from build123d import *

# Parameters (mm, degrees)
SKETCH1_W                                           = 65
SKETCH1_H                                           = 75
BOSS_EXTRUDE1_DEPTH                                 = 10
SKETCH2_W                                           = 5
SKETCH2_H                                           = 75
BOSS_EXTRUDE2_DEPTH                                 = 15
CUT_EXTRUDE1_DEPTH                                  = 109
CUT_EXTRUDE3_DEPTH                                  = 6.2
CUT_EXTRUDE4_DEPTH                                  = 48.4
CBORE_FOR_M6_HEX_SOCKET_HEAD_CAP_SCREW1_D           = 6.6
CBORE_FOR_M6_HEX_SOCKET_HEAD_CAP_SCREW1_CBORE_D     = 11
CBORE_FOR_M6_HEX_SOCKET_HEAD_CAP_SCREW1_CBORE_DEPTH = 6.2
BOSS_EXTRUDE3_START                                 = 5
SKETCH9_W                                           = 25
SKETCH9_H                                           = 75
BOSS_EXTRUDE3_DEPTH                                 = 5
CHAMFER1_SIZE                                       = 1.5


with BuildPart() as part:
    # Sketch1 → Boss-Extrude1 (new body)
    with BuildSketch(Plane.XY):
        Rectangle(SKETCH1_W, SKETCH1_H)
    extrude(amount=BOSS_EXTRUDE1_DEPTH)

    # Sketch2 → Boss-Extrude2 (add)
    with BuildSketch(Plane(origin=(0, 0, 0), x_dir=(-1, 0, 0), z_dir=(0, 0, -1))):
        with Locations((-30, 0)):
            Rectangle(SKETCH2_W, SKETCH2_H)
        with Locations((30, 0)):
            Rectangle(SKETCH2_W, SKETCH2_H)
    extrude(amount=BOSS_EXTRUDE2_DEPTH)

    # Sketch3 → Cut-Extrude1 (cut)
    with BuildSketch(Plane.ZY.offset(32.5)):
        with BuildLine():
            Line((-4.75, 30), (-4.75, -30))
            ThreePointArc((-4.75, -30), (-7.5, -32.75), (-10.25, -30))
            Line((-10.25, -30), (-10.25, 30))
            ThreePointArc((-10.25, 30), (-7.5, 32.75), (-4.75, 30))
        make_face()
    extrude(amount=-CUT_EXTRUDE1_DEPTH, mode=Mode.SUBTRACT)

    # Sketch4 → Cut-Extrude3 (cut)
    with BuildSketch(Plane(origin=(0, 0, 0), x_dir=(-1, 0, 0), z_dir=(0, 0, -1))):
        with BuildLine():
            ThreePointArc((-23.364355515, 19.605022095), (-22.686442931, 11.856445805), (-14.937866641, 12.534358389))
            ThreePointArc((-14.937866641, 12.534358389), (0, 19.5), (14.937866641, 12.534358389))
            ThreePointArc((14.937866641, 12.534358389), (22.686442931, 11.856445805), (23.364355515, 19.605022095))
            ThreePointArc((23.364355515, 19.605022095), (0, 30.5), (-23.364355515, 19.605022095))
        make_face()
    extrude(amount=-CUT_EXTRUDE3_DEPTH, mode=Mode.SUBTRACT)

    # Sketch5 → Cut-Extrude4 (cut)
    with BuildSketch(Plane(origin=(0, 0, 0), x_dir=(-1, 0, 0), z_dir=(0, 0, -1))):
        with BuildLine():
            ThreePointArc((-21.67905774, 18.190889354), (-21.27231019, 13.54174358), (-16.623164416, 13.94849113))
            ThreePointArc((-16.623164416, 13.94849113), (0, 21.7), (16.623164416, 13.94849113))
            ThreePointArc((16.623164416, 13.94849113), (21.27231019, 13.54174358), (21.67905774, 18.190889354))
            ThreePointArc((21.67905774, 18.190889354), (0, 28.3), (-21.67905774, 18.190889354))
        make_face()
    extrude(amount=-CUT_EXTRUDE4_DEPTH, mode=Mode.SUBTRACT)

    # CBORE for M6 Hex Socket Head Cap Screw1 (through all)
    with Locations(Plane(origin=(0, 0, 0), x_dir=(-1, 0, 0), z_dir=(0, 0, -1))):
        with Locations((0, 0)):
            CounterBoreHole(CBORE_FOR_M6_HEX_SOCKET_HEAD_CAP_SCREW1_D / 2, CBORE_FOR_M6_HEX_SOCKET_HEAD_CAP_SCREW1_CBORE_D / 2, CBORE_FOR_M6_HEX_SOCKET_HEAD_CAP_SCREW1_CBORE_DEPTH)

    # Sketch9 → Boss-Extrude3 (add)
    with BuildSketch(Plane.ZY.offset(32.5).offset(BOSS_EXTRUDE3_START)):
        with Locations((-2.5, 0)):
            Rectangle(SKETCH9_W, SKETCH9_H)
        with BuildLine():
            Line((-4.75, 30), (-4.75, -30))
            ThreePointArc((-4.75, -30), (-7.5, -32.75), (-10.25, -30))
            Line((-10.25, -30), (-10.25, 30))
            ThreePointArc((-10.25, 30), (-7.5, 32.75), (-4.75, 30))
        make_face(mode=Mode.SUBTRACT)
    boss_extrude3 = extrude(amount=-BOSS_EXTRUDE3_DEPTH)

    # Mirror1: Boss-Extrude3 across plane
    add(boss_extrude3.mirror(Plane.ZY))

    # Chamfer1
    chamfer1_edges = [part.edges().sort_by_distance(p)[0] for p in [
        (-37.5, 0, -15),
        (-37.5, -37.5, -2.5),
        (-37.5, 0, 10),
        (-37.5, 37.5, -2.5),
        (37.5, 0, -15),
        (37.5, 37.5, -2.5),
        (37.5, 0, 10),
        (37.5, -37.5, -2.5),
        (0, -37.5, 10),
        (32.5, -37.5, -15),
        (32.5, 37.5, -15),
        (-32.5, 37.5, -15),
        (-32.5, -37.5, -15),
        (0, 37.5, 10),
    ]]
    chamfer(chamfer1_edges, length=CHAMFER1_SIZE)


solid = part.part
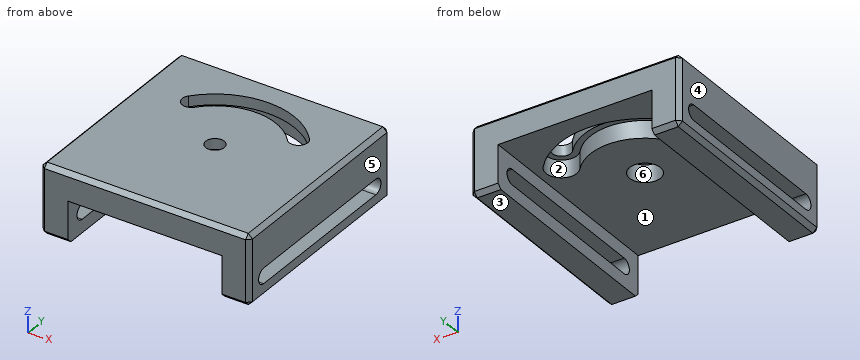
Check sheet for the modelled part. Datum: model origin and axes. Units: mm. Face numbers are marked on the shaded views. A direction names the side the tool comes from. Give positions to 0.01 mm unless a question says otherwise; leave off trailing zeros. Write each loop counter-clockwise with the first axis right and the second up, starting at its lowest first coordinate (ties: lowest second). Pieces come first, ordered by that corner, then holes. Notation, with made-up numbers: (77.5, -12.5) -> (109.5, -12.5) arc R25 cw to (109.5, 1.5) -> close; hole circle Ø2 at (64.5, -32). An arc over 180 degrees is marked (long way). One line per item, written item: value. Start each with the question number.
Item 1: Section check B-B on x = 30. Record the cut outline in (y, z), then the cut area to 3 significant figures.
Item 2: Section check C-C on z = 2.25. Record the cut outline in (x, y), then the cut area to 3 significant figures.
Item 3: Tool access check on the marked faces 1, 2 and 3. Record the directions out of +Z, -Z, +X, -X, +Y, -Y that give a thin tool (end or side, any length) a straight path to the whole face; none if there is none.
Item 4: Draft check along X on the marked faces 4, 5 and 6. Enter one of: +X half, -X half, draft (parallel to the pull), parting line (faces both ways), or undercut.
Item 5: Material ranges on probe 1 along Y at (x, z) = (0, 3.25); probe 2 along Y at (x, z) = (0, 8.25); probe 3 along X at (y, z) = (10.5, -12.75), recorded low to high. Write a range as from..to.
Item 6: Gauge pin test, flat ends, axial feed: pin 1 (9 mm diameter, centred on x = 0, y = 0, fed in from -Z); pin 2 (1.5 mm diameter, centred on x = 20.5, z = -2, fed in from -Y); pin 3 (10 mm diameter, centred on x = 8, y = 16.5, fed in from -Z). Record the tip position at first contact, or that the pin passes through.
Item 7: Section check A-A on y = 0. Record the cut outline in (x, z).
Item 8: Section check D-D on z = -7.5. Record the cut outline in (x, y), then the cut area to 4 significant figures.
Results list:
1. outline: (-37.5, -13.5) -> (-36, -15) -> (36, -15) -> (37.5, -13.5) -> (37.5, 8.5) -> (36, 10) -> (-36, 10) -> (-37.5, 8.5) -> close; hole (-30, -10.25) -> (30, -10.25) arc R2.75 ccw to (30, -4.75) -> (-30, -4.75) arc R2.75 ccw to start
1. area: 1,520 mm²
2. outline: (-37.5, -36) -> (-36, -37.5) -> (36, -37.5) -> (37.5, -36) -> (37.5, 36) -> (36, 37.5) -> (-36, 37.5) -> (-37.5, 36) -> close; hole (-23.36, 19.61) arc R5.5 ccw to (-14.94, 12.53) arc R19.5 cw to (14.94, 12.53) arc R5.5 ccw to (23.36, 19.61) arc R30.5 ccw to start; hole circle Ø11 at (0, 0)
2. area: 4,950 mm²
3. face 1: -Z, +Y, -Y
3. face 2: -Z
3. face 3: -Z, +X, -X, +Y, -Y
4. face 4: -X half
4. face 5: +X half
4. face 6: undercut
5. probe 1: -37.5..-5.5, 5.5..19.5, 30.5..37.5
5. probe 2: -37.5..-3.3, 3.3..21.7, 28.3..37.5
5. probe 3: -37.5..-27.5, 27.5..37.5
6. pin 1: z = 6.2
6. pin 2: through
6. pin 3: z = 0
7. outline: (-37.5, -13.5) -> (-36, -15) -> (-27.5, -15) -> (-27.5, -10.25) -> (-37.5, -10.25) -> close; (-37.5, -4.75) -> (-27.5, -4.75) -> (-27.5, 0) -> (-5.5, 0) -> (-5.5, 6.2) -> (-3.3, 6.2) -> (-3.3, 10) -> (-36, 10) -> (-37.5, 8.5) -> close; (3.3, 6.2) -> (5.5, 6.2) -> (5.5, 0) -> (27.5, 0) -> (27.5, -4.75) -> (37.5, -4.75) -> (37.5, 8.5) -> (36, 10) -> (3.3, 10) -> close; (27.5, -15) -> (36, -15) -> (37.5, -13.5) -> (37.5, -10.25) -> (27.5, -10.25) -> close
8. outline: (-37.5, -36) -> (-36, -37.5) -> (-27.5, -37.5) -> (-27.5, -32.75) -> (-37.5, -32.75) -> close; (-37.5, 32.75) -> (-27.5, 32.75) -> (-27.5, 37.5) -> (-36, 37.5) -> (-37.5, 36) -> close; (27.5, -37.5) -> (36, -37.5) -> (37.5, -36) -> (37.5, -32.75) -> (27.5, -32.75) -> close; (27.5, 32.75) -> (37.5, 32.75) -> (37.5, 36) -> (36, 37.5) -> (27.5, 37.5) -> close
8. area: 185.5 mm²
